Answer from the drawing. Dimensions are ordinates in mm from the lowest x, y and z of the part. A direction names the side the tool comes from. Round coordinates to 2 decimals unless told otherwise and drop trailing zeros. Write each loop counter-clockwise with the first axis right and the second up, starting at its lowest first coordinate (ties: lowest second). Pieces come first, ordered by that corner, then holes. Notation, with made-up numbers: M 16.25,48 L 70.25,48 A13 cw 70.25,73 Z; hole C -32.75,-0.5 d5. An arc over 180 degrees is marked long. One line per item, written item: value. Start each with the question number.
(1) Section D-D (x = 16) is taken. Determine the outline of the cut face in (y, z).
(2) Consider probe 1 along X at (y, z) = (10, 22); probe 2 along Y at (x, z) = (4, 4.3) (1 decimal); probe 3 along Z at (x, y) = (20, 13). Determine where each line is inside the solid, lowest interval first.
(3) For the marked faces 4, 5, 6 and 7, determine the directions among +Z, -Z, +X, -X, +Y, -Y from which every point of the face is accessible in a straight line to the end or side of a thin tool.
(4) Section C-C (y = 8.5) is taken. Determine the outline of the cut face in (x, z), plus the area to 3 significant figures.
(5) For a pull along X with two mould halves and no side action, classify the marked faces 1, 2 and 3 as released by +X, released by -X, zero draft, split by the parting line, or undercut.
(6) Section A-A (z = 6) is taken. Determine the outline of the cut face in (x, y).
(7) Given P1, Ø3, axis at y = 15.5, z = 10, coming from the -X side; P2, Ø1.1, axis at x = 23, y = 13.5, coming from the -Z side; P3, Ø3, axis at x = 4.5, y = 13, coming from the +Z side, each flat-ended and moving along its own axis, determine where each tip first touches the part or whether it passes through.
(8) Section B-B (x = 4) is taken. Determine the outline of the cut face in (y, z) (1 decimal), plus the area to 3 significant figures.
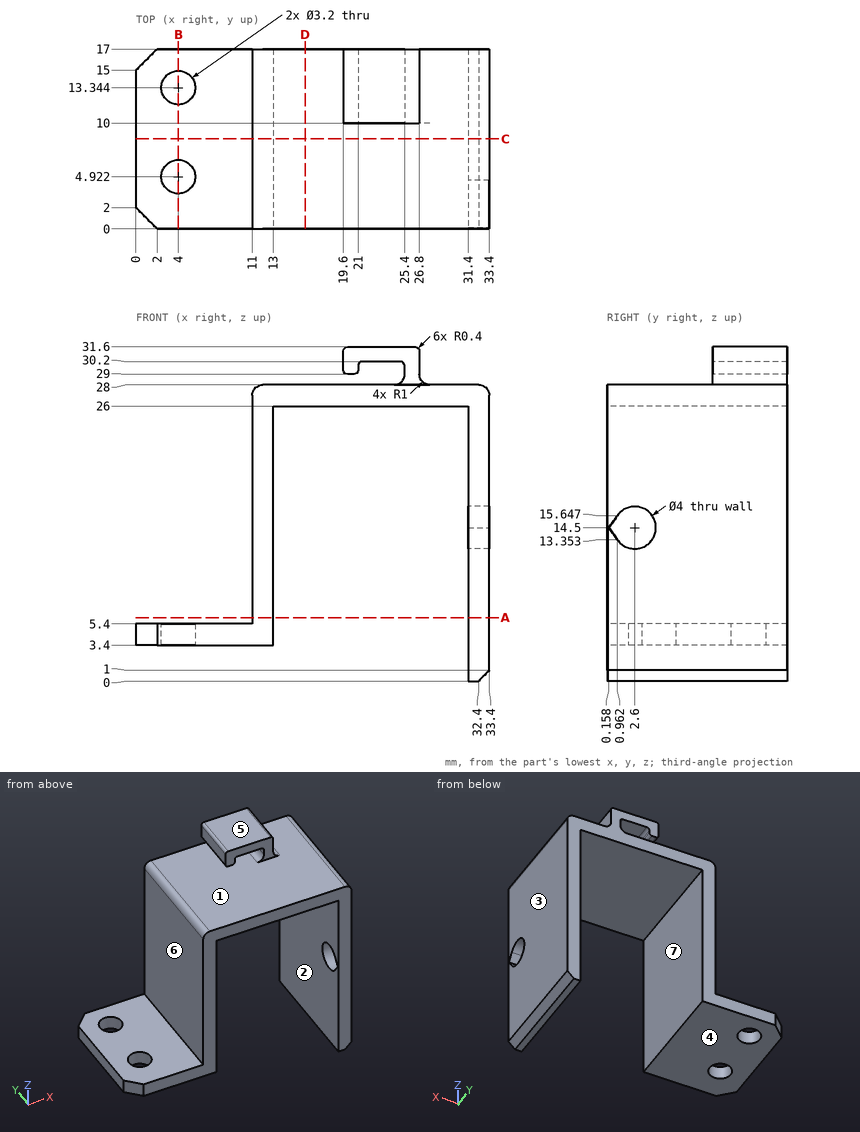
Recorded:
1. outline: M 0,26 L 17,26 L 17,28 L 0,28 Z
2. probe 1: x = 11 to 13, 31.4 to 33.4
2. probe 2: y = 0 to 3.3, 6.5 to 11.7, 14.9 to 17
2. probe 3: z = 26 to 28, 29 to 31.6
3. face 4: -Z, -X, +Y, -Y
3. face 5: +Z, +X, -X, +Y, -Y
3. face 6: +Z, -X, +Y, -Y
3. face 7: -Z, +Y, -Y
4. outline: M 0,3.4 L 13,3.4 L 13,26 L 31.4,26 L 31.4,0 L 32.4,0 L 33.4,1 L 33.4,27 A1 ccw 32.4,28 L 12,28 A1 ccw 11,27 L 11,5.4 L 0,5.4 Z
4. area: 163 mm2
5. face 1: zero draft
5. face 2: undercut
5. face 3: released by +X
6. outline: M 11,0 L 13,0 L 13,17 L 11,17 Z; M 31.4,0 L 33.4,0 L 33.4,17 L 31.4,17 Z
7. P1: stops at x = 11
7. P2: stops at z = 26
7. P3: stops at z = 5.4
8. outline: M 0,3.4 L 3.3,3.4 L 3.3,5.4 L 0,5.4 Z; M 6.5,3.4 L 11.7,3.4 L 11.7,5.4 L 6.5,5.4 Z; M 14.9,3.4 L 17,3.4 L 17,5.4 L 14.9,5.4 Z
8. area: 21.2 mm2
